Source: three-view drawing plus pictorial views. Frame: mm from the lowest corner of the part. A direction names the side the tool comes from. Round coordinates to 2 decimals unless told otherwise and drop trailing zeros. Write each loop counter-clockwise with the first axis right and the second up, starting at its lowest first coordinate (ties: lowest second). Pieces come first, ordered by that corner, then holes.
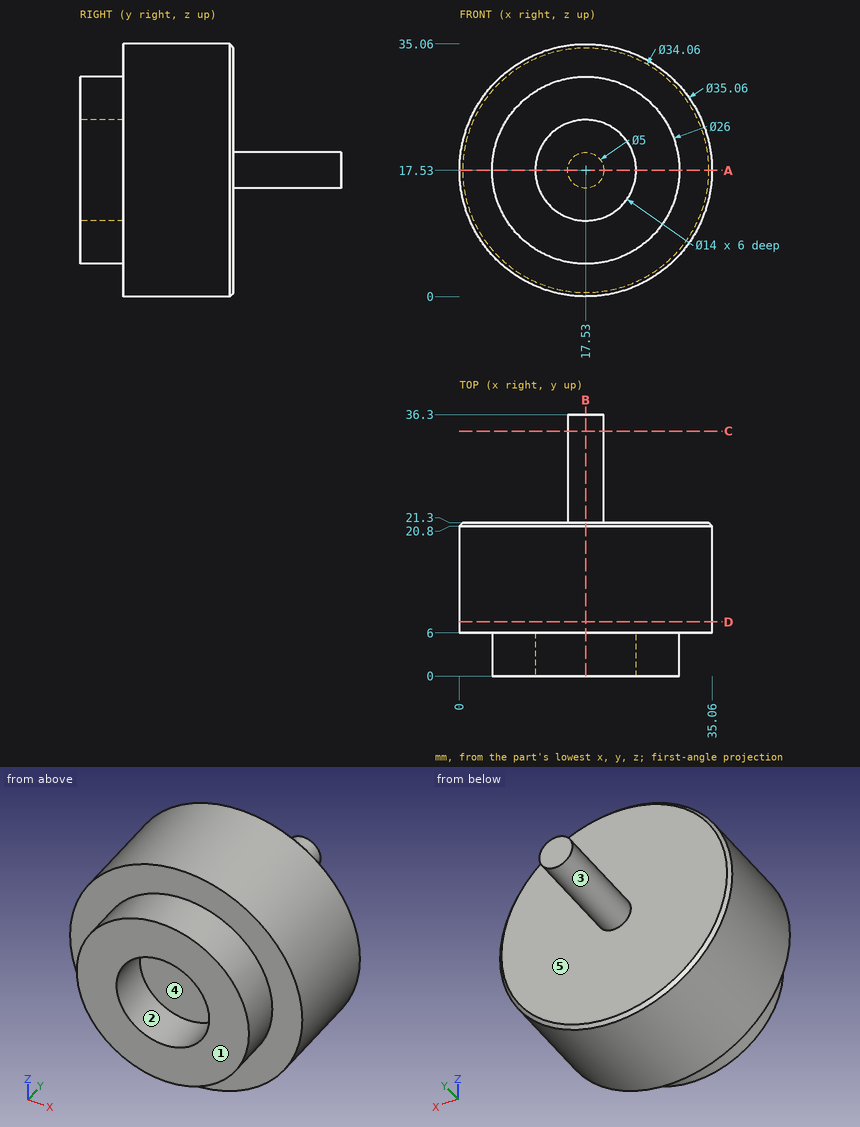
1) Line query: probe 1 along Z at (x, y) = (17.53, 3.8); probe 2 along Y at (x, z) = (17, 17.5); probe 3 along Y at (x, z) = (7, 14). Output: solid intervals per line, ascending.
2) Section C-C on y = 34. Output: boundary loops of the cut face in (x, z), plus the area to 3 significant figures.
3) Section D-D on y = 7.5. Output: boundary loops of the cut face in (x, z).
4) First-contact query: P1, Ø4, axis at x = 3.5, z = 14, coming from the +Y side; P2, Ø6, axis at x = 11, y = 26.5, coming from the +Z side; P3, Ø1.5, axis at y = 14.5, z = 14.5, coming from the +X side; P4, Ø6, axis at x = 5, y = 15.5, coming from the +Z side. Flat tips, straight axial feed; report the tip coordinate or a pass-through.
5) Section B-B on x = 17.53. Output: boundary loops of the cut face in (y, z).
6) Draft query along Z for the marked faces 3, 4 and 5. Return one class per face: pulls with the +Z half, pulls with the -Z half, needs draft (parallel to the pull), parting line crosses it, or undercut.
7) Reachability of the marked faces 1 and 2 from +Z, -Z, +X, -X, +Y, -Y: full face, straight path, thin tool, end or side. Return the list, or none.
8) Section A-A on z = 17.53. Output: boundary loops of the cut face in (x, y).
Filled in:
1. probe 1: z = 4.53 to 10.53, 24.53 to 30.53
1. probe 2: y = 6 to 36.3
1. probe 3: y = 0 to 21.3
2. outline: circle Ø5 at (17.53, 17.53)
2. area: 19.6 mm2
3. outline: circle Ø35.06 at (17.53, 17.53)
4. P1: stops at y = 21.3
4. P2: passes through
4. P3: stops at x = 34.91
4. P4: stops at z = 32.24
5. outline: (0, 4.53) - (6, 4.53) - (6, 0) - (20.8, 0) - (21.3, 0.5) - (21.3, 15.03) - (36.3, 15.03) - (36.3, 20.03) - (21.3, 20.03) - (21.3, 34.56) - (20.8, 35.06) - (6, 35.06) - (6, 30.53) - (0, 30.53) - (0, 24.53) - (6, 24.53) - (6, 10.53) - (0, 10.53) - close
6. face 3: parting line crosses it
6. face 4: undercut
6. face 5: needs draft
7. face 1: +Z, -Z, +X, -X, -Y
7. face 2: -Y
8. outline: (0, 6) - (4.53, 6) - (4.53, 0) - (10.53, 0) - (10.53, 6) - (24.53, 6) - (24.53, 0) - (30.53, 0) - (30.53, 6) - (35.06, 6) - (35.06, 20.8) - (34.56, 21.3) - (20.03, 21.3) - (20.03, 36.3) - (15.03, 36.3) - (15.03, 21.3) - (0.5, 21.3) - (0, 20.8) - close
